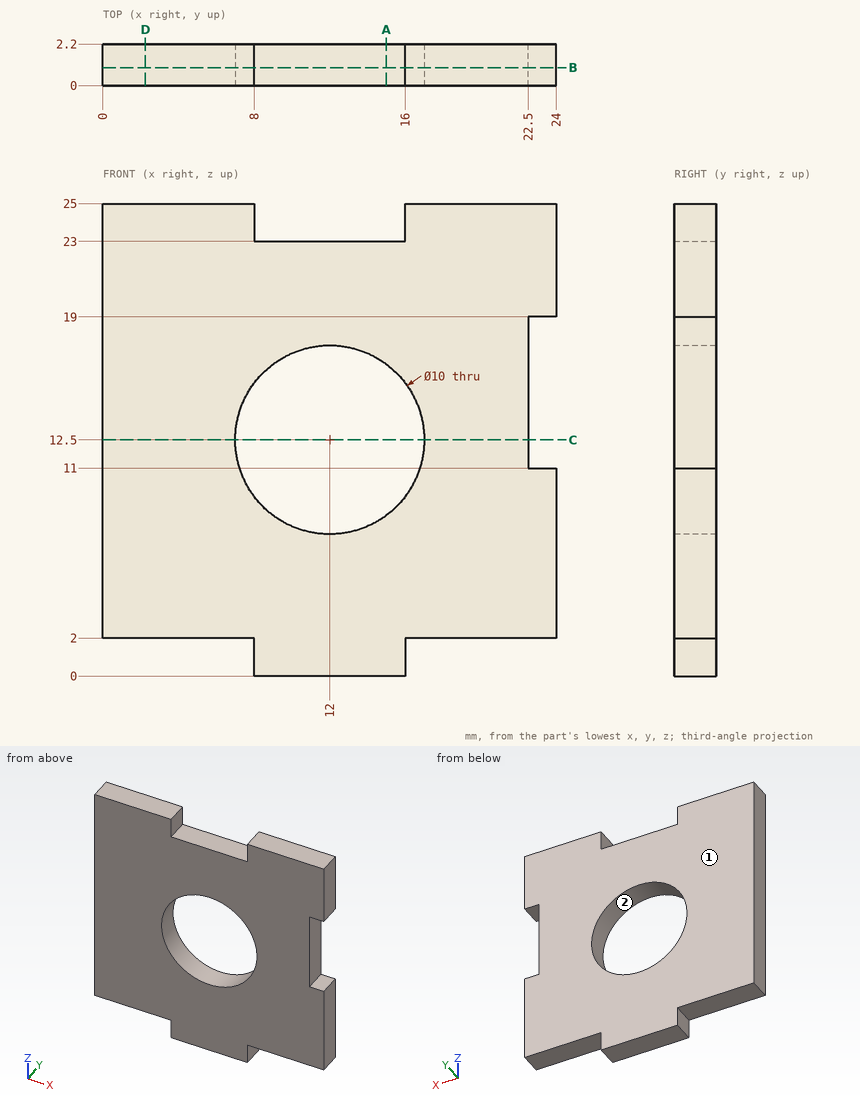
Part print with two shaded views. Sizes in mm from the minimum x, y, z corner. Round coordinates to 2 decimals unless told otherwise and drop trailing zeros. Write each loop counter-clockwise with the first axis right and the second up, starting at its lowest first coordinate (ties: lowest second). Pieces come first, ordered by that corner, then holes. Notation, with made-up numbers: (28.5, 78.25) -> (50.5, 78.25) arc R10 cw to (50.5, 87.25) -> close; hole circle Ø8 at (-36.5, 62.25). An arc over 180 degrees is marked (long way). Put each result on its own line as item: value.
Item 1: Slice it at D-D, the plane x = 2.25. Give the cut face in (y, z), plus the area to 3 significant figures.
Here are the results:
outline: (0, 2) -> (2.2, 2) -> (2.2, 25) -> (0, 25) -> close
area: 50.6 mm^2
Item 2: Slice it at C-C, the plane z = 12.5. Give the cut face in (x, y).
Here are the results:
outline: (0, 0) -> (7, 0) -> (7, 2.2) -> (0, 2.2) -> close; (17, 0) -> (22.5, 0) -> (22.5, 2.2) -> (17, 2.2) -> close
Item 3: Slice it at A-A, the plane x = 15. Give the cut face in (y, z), plus the area to 3 significant figures.
Here are the results:
outline: (0, 0) -> (2.2, 0) -> (2.2, 8.5) -> (0, 8.5) -> close; (0, 16.5) -> (2.2, 16.5) -> (2.2, 23) -> (0, 23) -> close
area: 33.0 mm^2
Item 4: Flat gauge pins, fed straight in: P1, Ø8, axis at x = 12, z = 12.5, coming from the -Y side; P2, Ø1.1, axis at y = 1, z = 16, coming from the +X side. Where does each tip first touch, or does it go through?
Here are the results:
P1: passes through
P2: stops at x = 22.5
Item 5: Slice it at B-B, the plane y = 0.95. Give the cut face in (x, z), plus the area to 3 significant figures.
Here are the results:
outline: (0, 2) -> (8, 2) -> (8, 0) -> (16, 0) -> (16, 2) -> (24, 2) -> (24, 11) -> (22.5, 11) -> (22.5, 19) -> (24, 19) -> (24, 25) -> (16, 25) -> (16, 23) -> (8, 23) -> (8, 25) -> (0, 25) -> close; hole circle Ø10 at (12, 12.5)
area: 461 mm^2
Item 6: Two-plate mould, pull along X, no slides. Class the marked faces 1 and 2: pulls with the +X half, pulls with the -X half, needs draft (parallel to the pull), parting line crosses it, or undercut.
Here are the results:
face 1: needs draft
face 2: undercut
Item 7: Wall check: probe 1 along X at (y, z) = (1, 12.5); probe 2 along Z at (x, y) = (17.75, 2.15); probe 3 along Z at (x, y) = (13.75, 1.35). Give the ranges that are in metal, low to high. Write a range as from..to.
Here are the results:
probe 1: x = 0..7, 17..22.5
probe 2: z = 2..25
probe 3: z = 0..7.82, 17.18..23
